Design review of the part built by this model. Coordinates are the model's own, in mm. Face numbers are marked on the shaded views. A direction names the side the tool comes from. Give positions to 0.01 mm unless a question says otherwise; leave off trailing zeros. Write each loop counter-clockwise with the first axis right and the second up, starting at its lowest first coordinate (ties: lowest second). Pieces come first, ordered by that corner, then holes. Notation, with made-up numbers: M 2.25,-18 L 27.25,-18 A13 ccw 27.25,-6 Z; hole C 75.5,71.5 d11. An arc over 180 degrees is marked long. Use a Markdown table: item, result. Add a question column.
```python
from build123d import *

# Parameters (mm, degrees)
SKETCH1_W                    = 48
SKETCH1_H                    = 32
BASE_FLANGE1_DEPTH           = 3.03784
EDGE_FLANGE1_STRIP_W         = 18.50136
EDGE_FLANGE1_STRIP_H         = 3.03784
EDGE_FLANGE1_STRIP_CUT_DEPTH = 48
EDGE_FLANGE1_DEPTH           = 48
M6_CLEARANCE_HOLE1_D         = 6.6
CUT_EXTRUDE1_DEPTH           = 63.481997407


# Sheet-metal steps are written as plain solids
with BuildPart() as part:
    # Sketch1 → Base-Flange1 (new body)
    with BuildSketch(Plane(origin=(0, 0, 0), x_dir=(1, 0, 0), z_dir=(0, 1, 0))):
        with Locations((0, 16)):
            Rectangle(SKETCH1_W, SKETCH1_H)
    extrude(amount=-BASE_FLANGE1_DEPTH)

    # Edge-Flange1 strip (across the edge) → Edge-Flange1 strip cut (cut)
    with BuildSketch(Plane(origin=(24, -3.03784, 0), x_dir=(0, 0, -1), z_dir=(-1, 0, 0))):
        with Locations((-3.03784, -1.51892)):
            Rectangle(EDGE_FLANGE1_STRIP_W, EDGE_FLANGE1_STRIP_H)
    extrude(amount=EDGE_FLANGE1_STRIP_CUT_DEPTH, mode=Mode.SUBTRACT)

    # Edge-Flange1 section (across the edge) → Edge-Flange1 (add)
    with BuildSketch(Plane(origin=(24, -3.03784, 0), x_dir=(0, 0, -1), z_dir=(-1, 0, 0))):
        with BuildLine():
            Line((0, 3.175), (0, 44.96216))
            Line((0, 44.96216), (3.03784, 44.96216))
            Line((3.03784, 44.96216), (3.03784, 3.175))
            ThreePointArc((3.03784, 3.175), (3.96777597, 0.92993597), (6.21284, 0))
            Line((6.21284, 0), (6.21284, -3.03784))
            ThreePointArc((6.21284, -3.03784), (1.819698706, -1.218141294), (0, 3.175))
        make_face()
    extrude(amount=EDGE_FLANGE1_DEPTH)

    # M6 Clearance Hole1 (through all)
    with Locations(Plane(origin=(0, -3.03784, 0), x_dir=(-1, 0, 0), z_dir=(0, -1, 0))):
        with Locations((12.5, 22), (-12.5, 22)):
            Hole(M6_CLEARANCE_HOLE1_D / 2)

    # Sketch13 → Cut-Extrude1 (cut, through all)
    with BuildSketch(Plane.XY):
        with BuildLine():
            Line((-9.75, -15), (-9.75, -23))
            ThreePointArc((-9.75, -23), (-12.5, -25.75), (-15.25, -23))
            Line((-15.25, -23), (-15.25, -15))
            ThreePointArc((-15.25, -15), (-12.5, -12.25), (-9.75, -15))
        make_face()
        with BuildLine():
            Line((15.25, -15), (15.25, -23))
            ThreePointArc((15.25, -23), (12.5, -25.75), (9.75, -23))
            Line((9.75, -23), (9.75, -15))
            ThreePointArc((9.75, -15), (12.5, -12.25), (15.25, -15))
        make_face()
    extrude(amount=-CUT_EXTRUDE1_DEPTH, mode=Mode.SUBTRACT)


solid = part.part
```
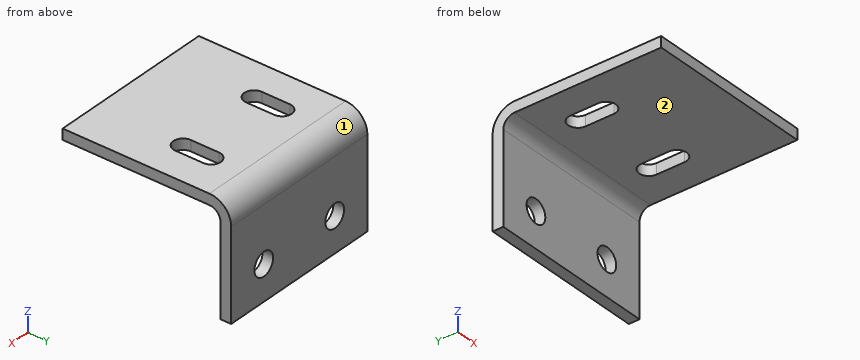
(1) Wall thickness on L1, parallel to X at y = -1.25, z = -22; L2, parallel to Z at x = -3, y = -11: over which ranges is each line inside the solid? List them lowest first.
(2) Add section A-A on x = 12.5. Give the boundary of the cut face in (y, z) (3 decimals), then the cut area to 3 significant figures.
(3) Machinability: for the marked faces 1 and 2, which of the approach directions +Z, -Z, +X, -X, +Y, -Y give a long, thin tool a straight path to every point of the face, cutting with its end or side? Answer none if there is none.
(4) Add section D-D on x = -8. Give the boundary of the cut face in (y, z) (3 decimals), then the cut area to 3 significant figures.
(5) For pin 1 (8 mm diameter, centred on x = 10, y = -14.5, fed in from -Z); pin 2 (10.5 mm diameter, centred on x = -12.5, z = -22, fed in from -Y), all flat-tipped, find the tip position at first contact; note any pin that passes through.
(6) Add section B-B on z = -22. Give the boundary of the cut face in (x, y), then the cut area to 3 significant figures.
(7) Add section C-C on y = -22. Give the boundary of the cut face in (x, z), then the cut area to 3 significant figures.
From the geometry:
| question | item | result |
|---|---|---|
| 1 | L1 | x = -24 to -15.8, -9.2 to 9.2, 15.8 to 24 |
| 1 | L2 | z = -3.04 to 0 |
| 2 | outline | M -48,-3.038 L -25.75,-3.038 L -25.75,0 L -48,0 Z; M -12.25,-3.038 L -6.213,-3.038 A3.175 cw -3.038,-6.213 L -3.038,-18.7 L 0,-18.7 L 0,-6.213 A6.213 ccw -6.213,0 L -12.25,0 Z; M -3.038,-32 L 0,-32 L 0,-25.3 L -3.038,-25.3 Z |
| 2 | area | 167 mm^2 |
| 3 | face 1 | +Z, +X, -X, +Y |
| 3 | face 2 | -Z, +X, -X, -Y |
| 4 | outline | M -48,-3.038 L -6.213,-3.038 A3.175 cw -3.038,-6.213 L -3.038,-32 L 0,-32 L 0,-6.213 A6.213 ccw -6.213,0 L -48,0 Z |
| 4 | area | 228 mm^2 |
| 5 | pin 1 | stops at z = -3.04 |
| 5 | pin 2 | stops at y = -3.04 |
| 6 | outline | M -24,-3.04 L -15.8,-3.04 L -15.8,0 L -24,0 Z; M -9.2,-3.04 L 9.2,-3.04 L 9.2,0 L -9.2,0 Z; M 15.8,-3.04 L 24,-3.04 L 24,0 L 15.8,0 Z |
| 6 | area | 106 mm^2 |
| 7 | outline | M -24,-3.04 L -15.25,-3.04 L -15.25,0 L -24,0 Z; M -9.75,-3.04 L 9.75,-3.04 L 9.75,0 L -9.75,0 Z; M 15.25,-3.04 L 24,-3.04 L 24,0 L 15.25,0 Z |
| 7 | area | 112 mm^2 |
